```python
from build123d import *

# Parameters (mm, degrees)
SKETCH3_R           = 0.9906
BOSS_EXTRUDE1_DEPTH = 0.9906
FILLET1_R           = 3.9624
FILLET2_R           = 1.9812
FILLET3_R           = 0.19812


with BuildPart() as part:
    # Sketch3 → Boss-Extrude1 (new, symmetric)
    with BuildSketch(Plane.XY):
        with BuildLine():
            Line((-7.963913355, -12.460220996), (-8.414612562, -8.997336074))
            ThreePointArc((-8.414612562, -8.997336074), (-12.230129097, 5.425677886), (0, 13.97))
            Line((0, 13.97), (0, 10.2108))
            ThreePointArc((0, 10.2108), (-10.208964753, 0.193585415), (-0.387101241, -10.203459672))
            Line((-0.387101241, -10.203459672), (-0.387101241, -14.7828))
            ThreePointArc((-0.387101241, -14.7828), (-4.333988291, -14.138513667), (-7.963913355, -12.460220996))
        make_face()
        with Locations((-3.663271004, -11.95047233)):
            Circle(SKETCH3_R, mode=Mode.SUBTRACT)
    extrude(amount=BOSS_EXTRUDE1_DEPTH, both=True)

    # Fillet1
    fillet1_edges = [part.edges().sort_by_distance(p)[0] for p in [
        (-8.414612562, -8.997336074, 0),
    ]]
    fillet(fillet1_edges, radius=FILLET1_R)

    # Fillet2
    fillet2_edges = [part.edges().sort_by_distance(p)[0] for p in [
        (-7.963913355, -12.460220996, 0),
    ]]
    fillet(fillet2_edges, radius=FILLET2_R)

    # Mirror1: part across plane


with BuildPart() as part_1:
    add(part.part)
    add(part.part.mirror(Plane(origin=(0, 13.97, 0.9906), x_dir=(0, 0, 1), z_dir=(-1, 0, 0))))

    # Fillet3
    fillet3_edges = [part_1.edges().sort_by_distance(p)[0] for p in [
        (-10.208964753, 0.193585415, 0.9906),
        (-8.159915946, -10.954262245, -0.9906),
        (-8.159915946, -10.954262245, 0.9906),
        (-8.594751987, -9.188846365, -0.9906),
        (-8.594751987, -9.188846365, 0.9906),
        (-3.835638548, -14.281768103, -0.9906),
        (-3.835638548, -14.281768103, 0.9906),
        (-7.758056172, -12.367660081, -0.9906),
        (-7.758056172, -12.367660081, 0.9906),
        (-12.002363858, 6.004215822, 0.9906),
        (3.835638548, -14.281768103, -0.9906),
        (8.159915946, -10.954262245, -0.9906),
        (8.159915946, -10.954262245, 0.9906),
        (3.835638548, -14.281768103, 0.9906),
        (8.594751987, -9.188846365, 0.9906),
        (8.594751987, -9.188846365, -0.9906),
        (7.758056172, -12.367660081, 0.9906),
        (7.758056172, -12.367660081, -0.9906),
        (-10.208964753, 0.193585415, -0.9906),
        (-12.002363858, 6.004215822, -0.9906),
    ]]
    fillet(fillet3_edges, radius=FILLET3_R)


solid = part_1.part
```
Input: part model. Units: mm. Frame: model coordinates. A direction names the side the tool comes from. Give positions to 0.01 mm unless a question says otherwise; leave off trailing zeros. Order: outer loops, then holes, each group sorted by start corner. A loop starts at its lowest first (then second) coordinate and runs counter-clockwise, first axis right, second up. Notation, with made-up numbers: (14.25, 55.25) - (22.25, 55.25) arc R14 ccw to (22.25, 76.25) - close; hole circle Ø2 at (87, 51.25). An arc over 180 degrees is marked (long way). One line per item, written item: value.
1. Line query: probe 1 along Y at (x, z) = (-3.5, 0); probe 2 along Y at (x, z) = (-3.75, -0.7); probe 3 along Y at (x, z) = (2.5, 0.2). Output: solid intervals per line, ascending.
Determined:
probe 1: -14.37 to -12.93, -10.97 to -9.59, 9.59 to 13.49
probe 2: -14.3 to -12.94, -10.96 to -9.5, 9.5 to 13.42
probe 3: -14.58 to -9.9, 9.9 to 13.73
2. Cut plane A-A, the plane z = 0.1. Output: boundary loops of the cut face in (x, y).
Determined:
outline: (-9.32, -8.15) arc R3.96 cw to (-8.23, -10.41) - (-8.09, -11.5) arc R1.98 ccw to (-7.07, -12.99) arc R14.79 ccw to (-0.39, -14.78) - (-0.39, -10.2) arc R10.21 cw (long way) to (0.39, -10.2) - (0.39, -14.78) arc R14.79 ccw to (7.07, -12.99) arc R1.98 ccw to (8.09, -11.5) - (8.23, -10.41) arc R3.96 cw to (9.32, -8.15) arc R13.03 ccw (long way) to start; hole circle Ø1.98 at (-3.66, -11.95); hole circle Ø1.98 at (3.66, -11.95)
3. Reachability of faces 1 (the face through (-0.387, -12, 0)), 2 (the face through (-11, 0, -0.991)) from +Z, -Z, +X, -X, +Y, -Y: full face, straight path, thin tool, end or side. Return the list, or none.
Determined:
face 1: +Z, -Z, -Y
face 2: -Z, +X, -X, +Y, -Y
4. Draft query along X for faces 3 (the face through (0.387, -12, 0)), 4 (the face through (3.878, -12.918, -0.014)), 5 (the face through (7.765, -12.357, 0.011)), 6 (the face through (-3.788, -14.294, 0.011)). Return one class per face: released by +X, released by -X, zero draft, split by the parting line, or undercut.
Determined:
face 3: undercut
face 4: undercut
face 5: released by +X
face 6: released by -X
5. Cut plane B-B, the plane x = 3. Give the number of separate pieces and of enclosed holes in the cut face, and give its area (3 significant figures).
Determined:
separate pieces: 3
enclosed holes: 0
area: 14.0 mm2
6. Pin query (flat end, axial travel): pin 1 Ø1.8 at (x, y) = (3.66, -11.95) entering from +Z; pin 2 Ø0.6 at (y, z) = (-12, 0) entering from -X. Return the tip coordinate at first contact, or that it passes through.
Determined:
pin 1: through
pin 2: x = -8.05
